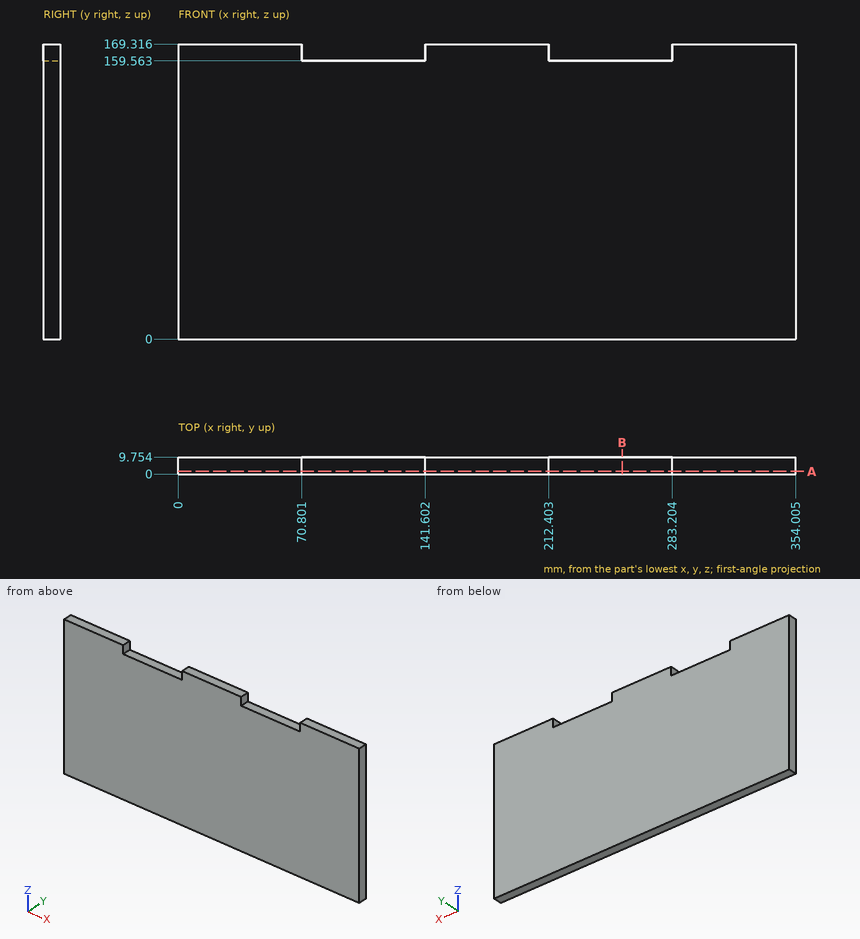
Verification items for this drawing (mm, ordinates from the low corner). Give positions to 0.01 mm unless a question says otherwise; leave off trailing zeros. Write each loop counter-clockwise with the first axis right and the second up, starting at its lowest first coordinate (ties: lowest second). Pieces come first, ordered by that corner, then holes. Notation, with made-up numbers: (-3.75, 0) - (44.25, 0) arc R12 cw to (44.25, 4) - close; hole circle Ø4 at (73, 18.5). An arc over 180 degrees is marked (long way). Answer as CSV lines item,"result". Start each with the question number.
1. Sectioned sample at A-A (y = 1.5). Record the boundary of the cut face in (x, z) (1 decimal).
2. Thickness scan on line 1 (Z direction, x = 278, y = 2.25). Record the ranges inside material, lowest first.
3. Depth check by flat-ended pin: pin 1 (1.5 mm diameter, centred on y = 1.5, z = 78.5, fed in from -X); pin 2 (3 mm diameter, centred on x = 99.5, y = 6.5, fed in from +Z). Enter the tip coordinate at first touch or a pass-through.
4. Sectioned sample at B-B (x = 254.5). Record the boundary of the cut face in (y, z), then the cut area to 3 significant figures.
Derived:
1,outline,"(0, 0) - (354, 0) - (354, 169.3) - (283.2, 169.3) - (283.2, 159.6) - (212.4, 159.6) - (212.4, 169.3) - (141.6, 169.3) - (141.6, 159.6) - (70.8, 159.6) - (70.8, 169.3) - (0, 169.3) - close"
2,line 1,"0 to 159.56"
3,pin 1,"x = 0"
3,pin 2,"z = 159.56"
4,outline,"(0, 0) - (9.75, 0) - (9.75, 159.56) - (0, 159.56) - close"
4,area,"1,560 mm²"
